Can you work these out from the model? Positions are in its coordinate system, mm. Face numbers are marked on the shaded views. A direction names the side the tool comes from. Give positions to 0.01 mm unless a question says otherwise; leave off trailing zeros. Order: outer loops, then holes, each group sorted by start corner. A loop starts at its lowest first (then second) coordinate and runs counter-clockwise, first axis right, second up. Notation, with made-up numbers: M 35,6 L 60,6 A21 ccw 60,27 Z; hole C -6.75,49.25 d7. An arc over 180 degrees is marked long. One line per question, with ' | ' between items. Start each with the question number.
1) If we section it at D-D, the plane z = 5.75: Please give me the cut outline in (x, y).
2) If we section it at A-A, the plane y = -25: Please give me the cut outline in (x, z), plus the area to 3 significant figures.
3) I'm going to push flat-ended pins straight in: pin 1 Ø1.5 at (x, y) = (5.5, -18.5) entering from -Z; pin 2 Ø3 at (x, y) = (2.5, -27) entering from +Z; pin 3 Ø1.8 at (x, z) = (9.5, -1.5) entering from -Y. Where does each tip first touch, or does it pass through?
4) If we section it at B-B, the plane z = 0: Please give me the cut outline in (x, y).
5) For the marked faces 1, 2, 3 and 4, which set-ups out of +Z, -Z, +X, -X, +Y, -Y let a thin tool reach every point of the face, with its end or its side?
6) If we section it at C-C, the plane x = 7.25: Please give me the cut outline in (y, z), plus the area to 3 significant figures.
7) Please list where these lines run through material, in increasing order: line 1 along Z through (x, y) = (6.5, -3.5); line 2 along X through (y, z) = (-16, 0.75); line 3 along Y through (x, z) = (9, 1.5). Write a range as [from, to].
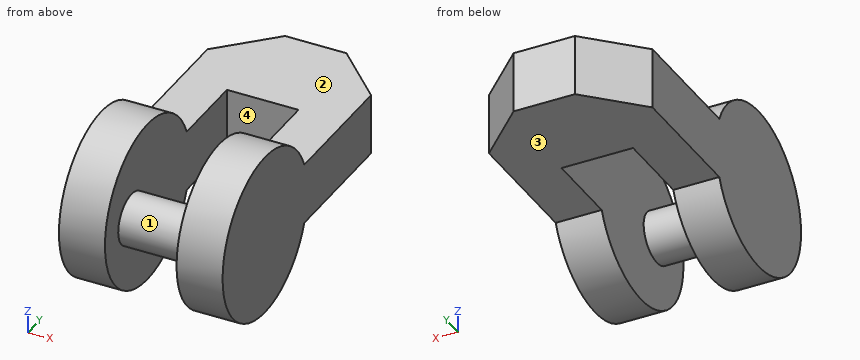
Autodesk Inventor part; units mm, degrees
ref_plane "작업 평면1" through (8, -10, 3) normal (1, 0, 0) x (0, 0, -1)
ref_plane "YZ Plane" through (0, 0, 0) normal (1, 0, 0) x (0, 1, 0)
ref_plane "XZ Plane" through (0, 0, 0) normal (0, 1, 0) x (-1, 0, 0)
sketch "스케치1" plane through (0, 0, 0) normal (0, 0, 1) x (1, 0, 0)
  line L0 (0, 0) -> (0, -28)
  line L1 (0, -28) -> (4.5, -28)
  line L2 (4.5, -26.5) -> (4.5, -10)
  line L3 (4.5, -10) -> (8, -10)
  line L4 (8, -10) -> (8, 0)
  line L5 (8, 0) -> (0, 0)
  line L6 (4.5, -28) -> (4.5, -26.5)
  dimension "d0" = 28
  dimension "d1" = 10
  dimension "d6" = 8
extrude "돌출1" add sketch "스케치1" along normal mid plane 6
mirror "미러1" about plane through (8, -10, 0) normal (1, 0, 0) of "돌출1"
chamfer "모따기1" distance 5 angle 45 1 edges at (0, 0, 0)
chamfer "모따기2" distance 5 angle 45 1 edges at (16, 0, 0)
sketch "스케치2" plane through (0, -28, -3) normal (-1, 0, 0) x (0, 0, 1)
  circle A0 centre (3, 3) radius 8
  line L0 (0, 0) -> (6, 0)
  point P0 (3, 28)
  dimension "d15" = 16
  dimension "d16" = 3
extrude "돌출2" add sketch "스케치2" against normal blind 4.5
ref_plane "작업 평면1" through (8, -10, 3) normal (1, 0, 0) x (0, 0, -1)
mirror "미러2" about plane through (8, -10, 3) normal (1, 0, 0) of "돌출2"
sketch "스케치3" plane through (4.5, -10, 3) normal (1, 0, 0) x (0, 0, -1)
  circle A0 centre (3, -18) radius 2.5
  line L0 (6, 10) -> (6, 5)
  point P0 (3, 10)
  dimension "d19" = 5
  dimension "d20" = 28
  dimension "d21" = 3
extrude "돌출3" add sketch "스케치3" along normal blind 7
ref_plane "작업 평면2" through (8, -10, 3) normal (1, 0, 0) x (0, 0, -1)
properties part number "2번부품"
Results found:
1) outline: M 0,-30.56 L 4.5,-30.56 L 4.5,-19.44 L 0,-19.44 Z; M 11.5,-30.56 L 16,-30.56 L 16,-19.44 L 11.5,-19.44 Z
2) outline: M 0,-8 L 4.5,-8 L 4.5,8 L 0,8 Z; M 11.5,-8 L 16,-8 L 16,8 L 11.5,8 Z | area: 144 mm²
3) pin 1: passes through | pin 2: stops at z = 7.98 | pin 3: stops at y = -30.43
4) outline: M 0,-33 L 4.5,-33 L 4.5,-30.5 L 11.5,-30.5 L 11.5,-33 L 16,-33 L 16,-5 L 11,0 L 5,0 L 0,-5 Z; hole M 4.5,-25.5 L 11.5,-25.5 L 11.5,-10 L 4.5,-10 Z
5) face 1: none | face 2: +Z, +X, -X, +Y | face 3: -Z, +X, -X, +Y | face 4: +Z, -Z
6) outline: C -28,0 d5; M -10,-3 L 0,-3 L 0,3 L -10,3 Z | area: 79.6 mm²
7) line 1: z = [-3, 3] | line 2: x = [0, 4.5], [11.5, 16] | line 3: y = [-30, -26], [-10, 0]
